Autodesk Inventor part; units mm, degrees
ref_plane "YZ Plane" through (0, 0, 0) normal (1, 0, 0) x (0, 1, 0)
ref_plane "XZ Plane" through (0, 0, 0) normal (0, 1, 0) x (-1, 0, 0)
ref_plane "XY Plane" through (0, 0, 0) normal (0, 0, 1) x (1, 0, 0)
sketch "Sketch1" plane through (0, 0, 0) normal (0, 0, 1) x (1, 0, 0)
  line L0 (38, 335) -> (0, 335)
  line L1 (0, 335) -> (0, 256.8)
  line L2 (0, 256.8) -> (0, 0) construction
  line L3 (0, 0) -> (38, 0) construction
  line L4 (38, 335) -> (38, 256.8)
  line L5 (38, 256.8) -> (0, 256.8)
  line L6 (38, 256.8) -> (38, 0) construction
  dimension "d0" = 670
  dimension "d1" = 38
  dimension "d5" = 513.6
revolve "Revolution1" add sketch "Sketch1" angle 360 about axis through (0, 0, 0) along (1, 0, 0)
sketch "Sketch2" plane through (0, 0, 0) normal (-1, 0, 0) x (0, 0, 1)
  circle A0 centre (0, 0) radius 256.8
  line L0 (0, 310) -> (0, 0) construction
  circle A1 centre (0, 0) radius 335
  circle A2 centre (0, 0) radius 310 construction
  line L1 (0, 0) -> (48.4947, 306.1834) construction
  circle A3 centre (48.4947, 306.1834) radius 13
  dimension "d6" = 26
  dimension "d7" = 310
  dimension "d8" = 9
extrude "Extrusion1" cut sketch "Sketch2" against normal through all contours A3
pattern_circular "Circular Pattern1" count 20 over 360 about axis through (19, 0, 0) along (1, 0, 0) of "Extrusion1"
equation "\"d6\" = dd2"
equation "\"d7\" = 0.5 * k"
equation "\"d0\" = D"
equation "\"d1\" = b"
equation "\"d5\" = dd5"
equation "\"b\" = 38"
equation "\"D\" = 670"
equation "\"dd2\" = 26"
equation "\"dd5\" = 513.6"
equation "\"Size_Designation\" = 1.2345"
properties part number "DIN 2576 Slip-On Flange for Welding Series 1 (ISO) - PN 10 500 x 508" material "Steel"
Model file for the job. Use its own axes, mm. Give positions to 0.01 mm unless a question says otherwise; leave off trailing zeros. Loops run counter-clockwise (first coordinate to the right, second up) from the corner with the lowest first, then second, coordinate; pieces in that order, holes last.
Item 1: Slice it at A-A (z = 0). Write the cut outline in (x, y).
Check values:
outline: (0, -335) - (38, -335) - (38, -256.8) - (0, -256.8) - close; (0, 256.8) - (38, 256.8) - (38, 335) - (0, 335) - close
Item 2: Drill centre lines: line 1 along Y through (x, z) = (7.5, -9); line 2 along Z through (x, y) = (34, 139); line 3 along Y through (x, z) = (22, 227). Where is each one in solid material? Low to high.
Check values:
line 1: y = -334.88 to -256.64, 256.64 to 334.88
line 2: z = -304.8 to -289.1, -263.33 to -215.93, 215.93 to 263.33, 289.1 to 304.8
line 3: y = -246.37 to -229.61, -208.8 to -120.07, 120.07 to 208.8, 229.61 to 246.37
Item 3: Drop flat-ended pins along their axis: P1, Ø2, axis at x = 10.5, y = 164.5, coming from the +Z side; P2, Ø4, axis at x = 24.5, z = -237.5, coming from the -Y side; P3, Ø3, axis at x = 18.5, z = -79, coming from the -Y side; P4, Ø5, axis at y = -264, z = 32.5, coming from the -X side. Give the stop position or say it passes through.
Check values:
P1: stops at z = 292.39
P2: stops at y = -238.25
P3: stops at y = -325.91
P4: stops at x = 0
